For this review, take the finished solid that the model builds, in its own axes (mm). A direction names the side the tool comes from. Coordinates: 2 decimals unless noted, no trailing zeros. Loops run counter-clockwise (first coordinate to the right, second up) from the corner with the lowest first, then second, coordinate; pieces in that order, holes last. Notation, with made-up numbers: (-21, -2) - (5, -2) arc R25 ccw to (5, 25) - close; hole circle Ø11 at (36.25, -16.75). An arc over 180 degrees is marked (long way). One line per item, written item: value. Start each with the question number.
1. To check wall thickness, follow line 1 (Y direction, x = 32, z = -0.1); line 2 (Y direction, x = 4, z = -1.65). State the ranges of each line that lie inside material, in increasing order. Write a range as from..to.
2. For faces 1 (the face through (55, 0, 0)), 2 (the face through (47.35, -0.54, -2.44)), list the 3-axis set-ups (+Z, -Z, +X, -X, +Y, -Y) from which the entire face can be reached by the end or side of a thin tool; tool diameter is ignored.
3. Insertion check: pin 1 (1.5 mm diameter, centred on x = 32.5, y = -1.5, fed in from +Z); pin 2 (1 mm diameter, centred on x = 9, y = -1.5, fed in from -Z); pin 3 (1.5 mm diameter, centred on y = 0.5, z = -0.5, fed in from -X). Each pin has a flat end and moves straight along its axis. Give the tip position at first contact, or say it passes through.
4. The part is to be moulded in two halves that separate along Z. For faces 3 (the face through (0, 0, 0)), 4 (the face through (20, -3, 0)), say which applies: released by +Z, released by -Z, zero draft, split by the parting line, or undercut.
5. Take a section at C-C, the plane x = 46. State the section outline as (y, z) points.
6. Take a section at D-D, the plane x = 12.5. State the section outline as (y, z) points.
Autodesk Inventor part; units mm, degrees
ref_plane "Startebene" through (0, 0, 0) normal (1, 0, 0) x (0, 1, 0)
ref_plane "XZ Plane" through (0, 0, 0) normal (0, 1, 0) x (-1, 0, 0)
ref_plane "XY Plane" through (0, 0, 0) normal (0, 0, 1) x (1, 0, 0)
sketch "Hauptskizze" plane through (0, 0, 0) normal (0, 0, 1) x (1, 0, 0)
  line L0 (0, 0) -> (55, 0)
  line L1 (0, 0) -> (0, 3)
  line L2 (40, 3) -> (40, 2.5)
  line L3 (0, 3) -> (40, 3)
  line L4 (55, 2.5) -> (55, 0)
  line L5 (40, 2.5) -> (55, 2.5)
  dimension "d3" = 6
  dimension "d14" = 5
revolve "Umdrehung1" add sketch "Hauptskizze" angle 360 about axis through (0, 0, 0) along (1, 0, 0)
chamfer "Fase4" distance 0.5 angle 45 1 edges at (0, -3, 0) measured on face at (13.3333, 2.9612, -0.4812)
chamfer "Fase5" distance 0.5 angle 45 1 edges at (55, -2.5, 0) measured on face at (45, 2.4919, -0.2012)
chamfer "Fase3" [suppressed]
chamfer "Fase2" distance 0.5 angle 45 1 edges at (40, -3, 0) measured on face at (13.6667, 2.9903, -0.2414)
properties part number "Welle" material "Steel"
Solutions:
1. line 1: -3..3
1. line 2: -2.51..2.51
2. face 1: +Z, -Z, +X, +Y, -Y
2. face 2: +X
3. pin 1: z = 2.9
3. pin 2: z = -2.83
3. pin 3: x = 0
4. face 3: zero draft
4. face 4: split by the parting line
5. outline: circle Ø5 at (0, 0)
6. outline: circle Ø6 at (0, 0)
